from build123d import *

# Parameters (mm, degrees)
Y_KSEKLIK_EKSTR_ZYON1_DEPTH = 5
IZIM2_R                     = 2.5
KES_EKSTR_ZYON3_DEPTH       = 2.5
IZIM3_R                     = 1.25
KES_EKSTR_ZYON4_DEPTH       = 18.853571071
IZIM5_R                     = 0.6
KES_EKSTR_ZYON5_DEPTH       = 2.5
Y_KSEKLIK_EKSTR_ZYON3_DEPTH = 3
BOSS_EXTRUDE1_START         = 6
BOSS_EXTRUDE1_DEPTH         = 6
CHAMFER1_SIZE               = 5


with BuildPart() as part:
    # Çizim1 → Yükseklik-Ekstrüzyon1 (new body)
    with BuildSketch(Plane(origin=(0, 0, 0), x_dir=(1, 0, 0), z_dir=(0, 1, 0))):
        with BuildLine():
            Line((-4.5, -8), (-4.5, -11.66190379))
            ThreePointArc((-4.5, -11.66190379), (0, 12.5), (4.5, -11.66190379))
            Line((4.5, -11.66190379), (4.5, -8))
            ThreePointArc((4.5, -8), (0, -3.5), (-4.5, -8))
        make_face()
    extrude(amount=Y_KSEKLIK_EKSTR_ZYON1_DEPTH)

    # Çizim2 → Kes-Ekstrüzyon3 (cut)
    with BuildSketch(Plane(origin=(0, 0, 0), x_dir=(1, 0, 0), z_dir=(0, 1, 0))):
        with Locations(Location((0, 0, 0), (0, 0, 270))):
            Circle(IZIM2_R)
    extrude(amount=KES_EKSTR_ZYON3_DEPTH, mode=Mode.SUBTRACT)

    # Çizim3 → Kes-Ekstrüzyon4 (cut, through all)
    with BuildSketch(Plane.XZ.offset(-2.5)):
        with Locations(Location((0, 0, 0), (0, 0, 270))):
            Circle(IZIM3_R)
    extrude(amount=-KES_EKSTR_ZYON4_DEPTH, mode=Mode.SUBTRACT)

    # Çizim5 → Kes-Ekstrüzyon5 (cut)
    with BuildSketch(Plane(origin=(0, 5, 0), x_dir=(1, 0, 0), z_dir=(0, 1, 0))):
        with Locations(Location((-6.449994102, -0.008722575, 0), (0, 0, 270))):
            Circle(IZIM5_R)
        with Locations(Location((6.449994102, 0.008722575, 0), (0, 0, 270))):
            Circle(IZIM5_R)
    extrude(amount=-KES_EKSTR_ZYON5_DEPTH, mode=Mode.SUBTRACT)

    # Çizim6 → Yükseklik-Ekstrüzyon3 (add)
    with BuildSketch(Plane(origin=(0, 5, 0), x_dir=(1, 0, 0), z_dir=(0, 1, 0))):
        with BuildLine():
            Line((-4.5, -11.66190379), (-4.5, -8))
            ThreePointArc((-4.5, -8), (0, -3.5), (4.5, -8))
            Line((4.5, -8), (4.5, -11.66190379))
            ThreePointArc((4.5, -11.66190379), (0, 12.5), (-4.5, -11.66190379))
        make_face()
        with BuildLine():
            Line((7, 1.991277425), (0.197348928, 2.523314182))
            ThreePointArc((0.197348928, 2.523314182), (0, 2.531019767), (-0.197348928, 2.523314182))
            Line((-0.197348928, 2.523314182), (-7, 1.991277425))
            ThreePointArc((-7, 1.991277425), (-9.021556758, -0.030279333), (-7, -2.051836091))
            Line((-7, -2.051836091), (-0.175036702, -2.524960042))
            ThreePointArc((-0.175036702, -2.524960042), (0, -2.531019767), (0.175036702, -2.524960042))
            Line((0.175036702, -2.524960042), (7, -2.051836091))
            ThreePointArc((7, -2.051836091), (9.021556758, -0.030279333), (7, 1.991277425))
        make_face(mode=Mode.SUBTRACT)
    extrude(amount=Y_KSEKLIK_EKSTR_ZYON3_DEPTH)

    # Sketch1 → Boss-Extrude1 (add)
    with BuildSketch(Plane.XZ.offset(-7.908623835).offset(BOSS_EXTRUDE1_START)):
        with BuildLine():
            Line((-4.5, 8), (4.5, 8))
            ThreePointArc((4.5, 8), (0, 3.5), (-4.5, 8))
        make_face()
    extrude(amount=-BOSS_EXTRUDE1_DEPTH)

    # Chamfer1
    # the kernel refuses this chamfer: 5 mm, written as the material it takes off along each edge
    with BuildSketch(Plane(origin=(-17.35841494, 1.908623835, 8), x_dir=(0, -0.027495876610586226, -0.9996219169112968), z_dir=(1, 0, 0))) as chamfer1_piece_1_section:
        Polygon((CHAMFER1_SIZE * 0.999621916911, CHAMFER1_SIZE * 0.0274958766106), (-CHAMFER1_SIZE * 0.0274958766106, CHAMFER1_SIZE * 0.999621916911), (0, 0), align=None)
    chamfer1_piece_1 = extrude(amount=34.71682988, mode=Mode.PRIVATE)
    chamfer1_piece_1 = chamfer1_piece_1 & Plane(origin=(0, 3.682638029, 8), x_dir=(1, 0, 0), z_dir=(0, -1, 0)) * Cylinder(4.5, 90, mode=Mode.PRIVATE)
    add(chamfer1_piece_1, mode=Mode.SUBTRACT)


solid = part.part
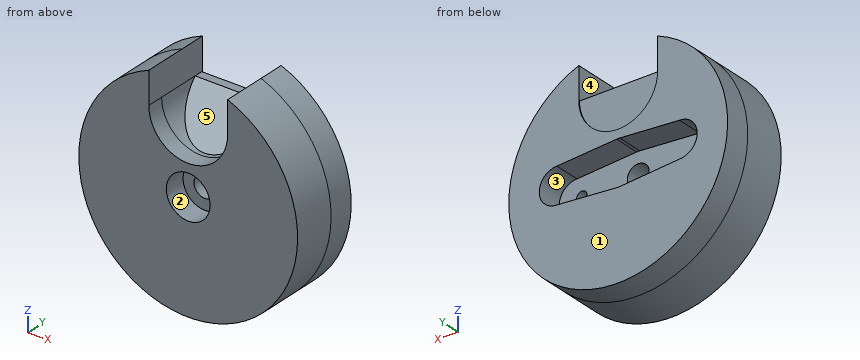
Can you work these out from the model? Positions are in its coordinate system, mm. Face numbers are marked on the shaded views. A direction names the side the tool comes from. Give positions to 0.01 mm unless a question says otherwise; leave off trailing zeros. Order: outer loops, then holes, each group sorted by start corner. A loop starts at its lowest first (then second) coordinate and runs counter-clockwise, first axis right, second up. Notation, with made-up numbers: M -30.5,69 L -14.5,69 A15 ccw -14.5,76 Z; hole C -38,59 d5. An arc over 180 degrees is marked long. Use one line per item in the form item = value. Start each with the question number.
Item 1: For the marked faces 3, 4 and 5, which set-ups out of +Z, -Z, +X, -X, +Y, -Y let a thin tool reach every point of the face, with its end or its side?
Item 2: If we section it at C-C (y = 1): Write out the boundary of the cut face in (x, z).
Item 3: If we section it at D-D (x = 5.5): Write out the boundary of the cut face in (y, z).
Item 4: Will these pins go through, and if not, where does the flat tip stop? pin 1 Ø12 at (x, z) = (8.5, 5.5) entering from -Y; pin 2 Ø1.5 at (x, y) = (-7, 5) entering from +Z; pin 3 Ø1.1 at (y, z) = (5, 9.5) entering from -X; pin 4 Ø2.5 at (x, z) = (1, 0.5) entering from -Y.
Item 5: We'd pull the mould along X, two halves only. Please class the marked faces 1 and 2: +X half, -X half, draft (parallel to the pull), parting line (faces both ways), or undercut.
Item 6: If we section it at A-A (z = 10.25): Write out the boundary of the cut face in (x, y).
Item 7: If we section it at B-B (y = 3.5): Write out the boundary of the cut face in (x, z).
Item 8: If I drill on line 1 along X through (y, z) = (3.4, 0); line 2 along X through (y, z) = (1.9, 0); line 3 along Z through (x, y) = (0.25, 1), over which ranges is the centre line in solid material (lowest first)?
Outcome:
q1.face_3 = +Y
q1.face_4 = +Z, +Y, -Y
q1.face_5 = +Z, -Y
q2.outline = M -4.5,8 L -4.5,11.66 A12.5 ccw long 4.5,11.66 L 4.5,8 A4.5 cw Z; hole C 0,0 d5
q3.outline = M 0,-11.22 L 8,-11.22 L 8,-2.11 L 5,-2.11 L 5,2.16 L 8,2.16 L 8,11.22 L 0,11.22 Z
q4.pin_1 = 0
q4.pin_2 = 10.83
q4.pin_3 = -8.73
q4.pin_4 = 2.5
q5.face_1 = draft
q5.face_2 = undercut
q6.outline = M -7.15,0 L -4.5,0 L -4.5,8 L -7.15,8 Z; M 4.5,0 L 7.15,0 L 7.15,8 L 4.5,8 Z
q7.outline = M -4.5,8 L -4.5,11.66 A12.5 ccw long 4.5,11.66 L 4.5,8 A4.5 cw 2.94,4.59 L -2.94,4.59 A4.5 cw Z; hole C -6.45,0.01 d1.2; hole C 0,0 d2.5; hole C 6.45,-0.01 d1.2
q8.line_1 = -12.5 to -7.05, -5.85 to -1.25, 1.25 to 5.85, 7.05 to 12.5
q8.line_2 = -12.5 to -2.5, 2.5 to 12.5
q8.line_3 = -12.5 to -2.49, 2.49 to 3.51
